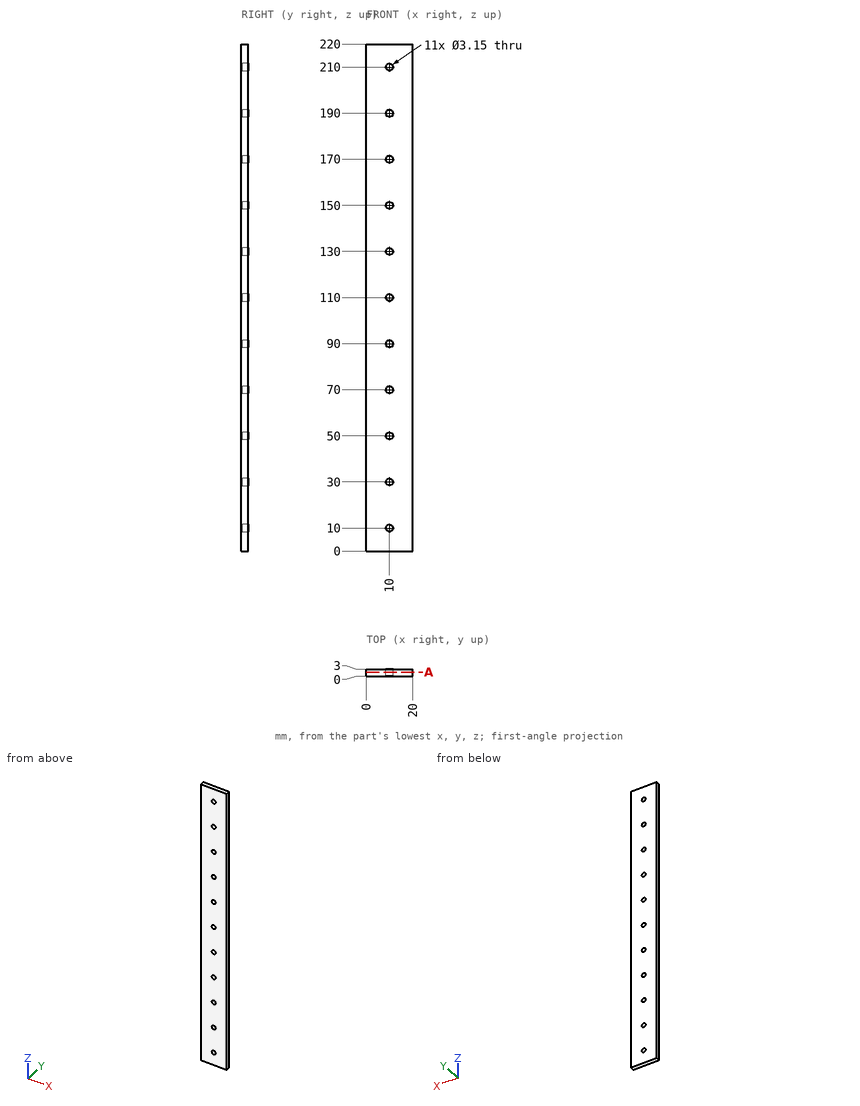
Source: three-view drawing plus pictorial views. Frame: mm from the lowest corner of the part. Give positions to 0.01 mm unless a question says otherwise; leave off trailing zeros. Put each result on its own line as item: value.
Q1. Section A-A, the plane y = 1.7. Count the separate pieces of the cut face and the enclosed holes in it, then the cut area to 3 significant figures.
Here are the results:
separate pieces: 1
enclosed holes: 11
area: 4,310 mm^2
Q2. Pin query (flat end, axial travel): pin 1 (2.5 mm diameter, centred on x = 10, z = 10, fed in from +Y). Return the tip coordinate at first contact, or that it passes through.
Here are the results:
pin 1: passes through
Q3. Material intervals for L1, parallel to X at y = 1.2, z = 50 (3 decimals); L2, parallel to X at y = 0.4, z = 149, sorted ascending.
Here are the results:
L1: x = 0 to 8.425, 11.575 to 20
L2: x = 0 to 8.78, 11.22 to 20
